The listing builds one solid part. Answer for the finished solid, in the listing's coordinates (mm). A direction names the side the tool comes from. Coordinates: 2 decimals unless noted, no trailing zeros. Order: outer loops, then holes, each group sorted by start corner. A loop starts at its lowest first (then second) coordinate and runs counter-clockwise, first axis right, second up. Notation, with made-up numbers: (66.25, 81) - (91.25, 81) arc R12 ccw to (91.25, 88) - close; hole circle Ø7 at (-31, -12). An arc over 180 degrees is marked (long way). Use one line per item in the form item = value. Start each with the question number.
Item 1: This flat-tipped pin is pushed along its axis until it touches: pin 1 Ø5.5 at (x, y) = (59, -12) entering from +Z (3 decimals). Where does it stop, or does it pass through?
Item 2: A tool of negligible diameter and unlimited length cuts with its end or side. For faces 1 (the flat face through (-27.758, -13, -1)), 2 (the flat face through (-18, -13, 30.755)), from which of +Z, -Z, +X, -X, +Y, -Y can it reach the whole face along a straight path? Write none if from no direction.
Item 3: Section A-A, the plane z = 0 is taken. Write down the section's boundary in (x, y), and give its area (3 significant figures).
Item 4: Section C-C, the plane y = -12.7 is taken. Write down the section's boundary in (x, z), and give its area (3 significant figures).
Item 5: Section B-B, the plane x = 23 is taken. Write down the section's boundary in (y, z).
Item 6: The mould has two halves that part along Y. Classify faces 3 (the flat face through (19, -25.4, -25)), 4 (the cylindrical face through (41.1, -12.5, 7.1)), 5 (the cylindrical face through (-23.353, -12.449, 34.374)): released by +Y, released by -Y, zero draft, split by the parting line, or undercut.
Item 7: Consider line 1 along X through (y, z) = (-23.75, 0.5); line 2 along X through (y, z) = (-14.75, -9); line 3 along Z through (x, y) = (31, -0.75). Determine where each line is inside the solid, lowest interval first. Write a range as [from, to].
from build123d import *

# Parameters (mm, degrees)
F0_W     = 95.25
F0_H     = 76.2
F0_R     = 23.749
F1_DEPTH = 25.4
F2_R     = 3.5687
F3_DEPTH = 7.1374
F4_R     = 5.715
F5_DEPTH = 7.1374


with BuildPart() as f1:
    # F0 (on Front) → F1 (new body)
    with BuildSketch(Plane.XZ):
        with Locations((19.8670865009, -0.2076110487)):
            Rectangle(F0_W, F0_H)
        with Locations((18.436120823, 0)):
            Circle(F0_R, mode=Mode.SUBTRACT)
    extrude(amount=F1_DEPTH)

    # F2 (on face) → F3 (cut)
    with BuildSketch(Plane.XY.offset(37.8923889513)):
        with Locations((57.6765805199, -11.9477792656)):
            Circle(F2_R)
    extrude(amount=F3_DEPTH, mode=Mode.SUBTRACT)

    # F4 (on face) → F5 (cut)
    with BuildSketch(Plane.XY.offset(37.8923889513)):
        with Locations((-17.6432492146, -12.7)):
            Circle(F4_R)
        with Locations((58.5567507854, -12.7)):
            Circle(F4_R)
    extrude(amount=-F5_DEPTH, mode=Mode.SUBTRACT)


solid = f1.part
Response:
q1.pin_1 = 30.755
q2.face_1 = +Z, -Z, -X, +Y, -Y
q2.face_2 = +Z
q3.outline = (-27.76, -25.4) - (-5.31, -25.4) - (-5.31, 0) - (-27.76, 0) - close; (42.19, -25.4) - (67.49, -25.4) - (67.49, 0) - (42.19, 0) - close
q3.area = 1,210 mm2
q4.outline = (-27.76, -38.31) - (67.49, -38.31) - (67.49, 37.89) - (64.27, 37.89) - (64.27, 30.75) - (52.84, 30.75) - (52.84, 37.89) - (-11.93, 37.89) - (-11.93, 30.75) - (-23.36, 30.75) - (-23.36, 37.89) - (-27.76, 37.89) - close; hole circle Ø47.5 at (18.44, 0)
q4.area = 5,320 mm2
q5.outline = (-25.4, -38.31) - (0, -38.31) - (0, -23.31) - (-25.4, -23.31) - close; (-25.4, 23.31) - (0, 23.31) - (0, 37.89) - (-25.4, 37.89) - close
q6.face_3 = released by -Y
q6.face_4 = zero draft
q6.face_5 = undercut
q7.line_1 = [-27.76, -5.31], [42.18, 67.49]
q7.line_2 = [-27.76, -3.54], [40.41, 67.49]
q7.line_3 = [-38.31, -20.15], [20.15, 37.89]
